from build123d import *

# Parameters (mm, degrees)
BOSS_EXTRUDE1_DEPTH     = 6
SKETCH2_R               = 7.5
BOSS_EXTRUDE2_DEPTH     = 30
BOSS_EXTRUDE3_DEPTH     = 6
SKETCH4_R               = 6.75
CUT_EXTRUDE1_DEPTH      = 49.476798574
CUT_EXTRUDE2_DEPTH      = 49.476798574
CUT_EXTRUDE2_DEPTH_BACK = 49.476798574
SKETCH5_W               = 23
SKETCH5_H               = 3
SKETCH6_R               = 2
CUT_EXTRUDE3_DEPTH      = 50.487372127


with BuildPart() as part:
    # Sketch1 → Boss-Extrude1 (new body)
    with BuildSketch(Plane.XY):
        with BuildLine():
            Line((-11, 0), (-11, -7))
            Line((-11, -7), (-19, -7))
            Line((-19, -7), (-19, -15))
            Line((-19, -15), (-11, -15))
            Line((-11, -15), (11, -15))
            Line((11, -15), (19, -15))
            Line((19, -15), (19, -7))
            Line((19, -7), (11, -7))
            Line((11, -7), (11, 0))
            ThreePointArc((11, 0), (0, 11), (-11, 0))
        make_face()
    extrude(amount=BOSS_EXTRUDE1_DEPTH)

    # Sketch2 → Boss-Extrude2 (add)
    with BuildSketch(Plane.XY.offset(6)):
        Circle(SKETCH2_R)
    extrude(amount=BOSS_EXTRUDE2_DEPTH)

    # Sketch3 → Boss-Extrude3 (add)
    with BuildSketch(Plane.XY.offset(36)):
        with BuildLine():
            Line((-11, 0), (-11, -7))
            Line((-11, -7), (-19, -7))
            Line((-19, -7), (-19, -15))
            Line((-19, -15), (19, -15))
            Line((19, -15), (19, -7))
            Line((19, -7), (11, -7))
            Line((11, -7), (11, 0))
            ThreePointArc((11, 0), (0, 11), (-11, 0))
        make_face()
    extrude(amount=BOSS_EXTRUDE3_DEPTH)

    # Sketch4 → Cut-Extrude1 (cut, through all)
    with BuildSketch(Plane.XY.offset(42)):
        Circle(SKETCH4_R)
    extrude(amount=-CUT_EXTRUDE1_DEPTH, mode=Mode.SUBTRACT)

    # Sketch5 → Cut-Extrude2 (cut, two sides: drawn at the far end of the back side and taken through both)
    with BuildSketch(Plane(origin=(0, 0, 0), x_dir=(-1, 0, 0), z_dir=(0, 0, -1)).offset(-CUT_EXTRUDE2_DEPTH_BACK)):
        with Locations((0, -13.5)):
            Rectangle(SKETCH5_W, SKETCH5_H)
    extrude(amount=CUT_EXTRUDE2_DEPTH + CUT_EXTRUDE2_DEPTH_BACK, mode=Mode.SUBTRACT)

    # Sketch6 → Cut-Extrude3 (cut, through all)
    with BuildSketch(Plane(origin=(0, -7, 0), x_dir=(1, 0, 0), z_dir=(0, 1, 0))):
        with Locations(Location((-15, -3, 0), (0, 0, 270))):
            Circle(SKETCH6_R)
        with Locations(Location((15, -3, 0), (0, 0, 270))):
            Circle(SKETCH6_R)
        with Locations(Location((15, -39, 0), (0, 0, 270))):
            Circle(SKETCH6_R)
        with Locations(Location((-15, -39, 0), (0, 0, 270))):
            Circle(SKETCH6_R)
    extrude(amount=-CUT_EXTRUDE3_DEPTH, mode=Mode.SUBTRACT)


solid = part.part
Here's how the part is built. I have some questions about the finished solid (model axes, mm). A direction names the side the tool comes from. Give positions to 0.01 mm unless a question says otherwise; leave off trailing zeros. Loops run counter-clockwise (first coordinate to the right, second up) from the corner with the lowest first, then second, coordinate; pieces in that order, holes last. Notation, with made-up numbers: (11, 25.5) -> (31, 25.5) arc R14 ccw to (31, 40.5) -> close; hole circle Ø2 at (31, 52). An arc over 180 degrees is marked (long way). One line per item, written item: value.
Q1. Suppose I cut it at C-C on x = 10.5. Please give me the cut outline in (y, z).
Answers follow:
outline: (-12, 0) -> (3.28, 0) -> (3.28, 6) -> (-12, 6) -> close; (-12, 36) -> (3.28, 36) -> (3.28, 42) -> (-12, 42) -> close
Q2. I'm going to push flat-ended pins straight in: pin 1 Ø4.5 at (x, z) = (15, 3) entering from +Y; pin 2 Ø1.5 at (y, z) = (-3.5, 11) entering from -X; pin 3 Ø10 at (x, z) = (2.5, 20) entering from +Y; pin 4 Ø3 at (x, z) = (-15, 3) entering from +Y. Where does each tip first touch, or does it pass through?
Answers follow:
pin 1: y = -7
pin 2: x = -6.98
pin 3: y = 7.5
pin 4: through
Q3. Suppose I cut it at D-D on y = 9. Please give me the cut outline in (x, z), then the cut area to 3 significant figures.
Answers follow:
outline: (-6.32, 0) -> (6.32, 0) -> (6.32, 6) -> (-6.32, 6) -> close; (-6.32, 36) -> (6.32, 36) -> (6.32, 42) -> (-6.32, 42) -> close
area: 152 mm^2
Q4. On a 3-axis mill with a long thin cutter (end or side, diameter ignored), from which of +Z, -Z, +X, -X, +Y, -Y can I reach the whole of each face in a straight line? I mean faces 1 (the face through (11, -4, 3)), 2 (the face through (0, -8, 36)), 3 (the face through (11.5, -14, 39)), 4 (the face through (17, -15, 2)), 5 (the face through (-19, -11, 3)). Say none if no direction works.
Answers follow:
face 1: +Z, -Z, +X, +Y
face 2: none
face 3: +Z, -Z, -Y
face 4: +Z, -Z, +X, -X, -Y
face 5: +Z, -Z, -X, +Y, -Y
Q5. Suppose I cut it at A-A on z = 39. Please give me the cut outline in (x, y), then the cut area to 3 significant figures.
Answers follow:
outline: (-19, -15) -> (-17, -15) -> (-17, -7) -> (-19, -7) -> close; (-13, -15) -> (-11.5, -15) -> (-11.5, -12) -> (11.5, -12) -> (11.5, -15) -> (13, -15) -> (13, -7) -> (11, -7) -> (11, 0) arc R11 ccw to (-11, 0) -> (-11, -7) -> (-13, -7) -> close; (17, -15) -> (19, -15) -> (19, -7) -> (17, -7) -> close; hole circle Ø13.5 at (0, 0)
area: 372 mm^2
Q6. If I drill on line 1 along X through (y, z) = (-8.25, 39); line 2 along X through (y, z) = (-12.75, 3); line 3 along Z through (x, y) = (16, -11.5), over which ranges is the centre line in solid material (lowest first)?
Answers follow:
line 1: -19 to -17, -13 to 13, 17 to 19
line 2: -19 to -17, -13 to -11.5, 11.5 to 13, 17 to 19
line 3: 0 to 1.27, 4.73 to 6, 36 to 37.27, 40.73 to 42
Q7. We'd pull the mould along X, two halves only. Please class faces 6 (the face through (-13, -11, 39)), 7 (the face through (-11, -3, 39)), 8 (the face through (19, -11, 39)): pulls with the +X half, pulls with the -X half, needs draft (parallel to the pull), parting line crosses it, or undercut.
Answers follow:
face 6: undercut
face 7: pulls with the -X half
face 8: pulls with the +X half
Q8. Suppose I cut it at B-B on y = -10.5. Please give me the cut outline in (x, z), then the cut area to 3 significant figures.
Answers follow:
outline: (-19, 0) -> (19, 0) -> (19, 6) -> (-19, 6) -> close; (-19, 36) -> (19, 36) -> (19, 42) -> (-19, 42) -> close; hole circle Ø4 at (-15, 3); hole circle Ø4 at (-15, 39); hole circle Ø4 at (15, 3); hole circle Ø4 at (15, 39)
area: 406 mm^2
